from build123d import *

# Parameters (mm, degrees)
SKETCH050_R      = 14.2875
PAD049_DEPTH     = 12.7
SKETCH049_R      = 23.8125
SKETCH049_R_2    = 6.35
PAD050_DEPTH     = 25.4
CHAMFER003_SIZE2 = 11.11
CHAMFER003_SIZE  = 4.76


with BuildPart() as body048:
    # Sketch050 → Pad049 (new body)
    with BuildSketch(Plane.XZ):
        Circle(SKETCH050_R)
    extrude(amount=PAD049_DEPTH)


with BuildPart() as chamfer003:
    # Sketch049 → Pad050 (new body)
    with BuildSketch(Plane.XZ):
        Circle(SKETCH049_R)
        Circle(SKETCH049_R_2, mode=Mode.SUBTRACT)
    extrude(amount=PAD050_DEPTH)

    # Cut047: cut Body048
    add(body048.part, mode=Mode.SUBTRACT)

    # Chamfer003
    chamfer003_edges = [chamfer003.edges().sort_by_distance(p)[0] for p in [
        (-23.8125, -25.4, 0),
    ]]
    chamfer003_side = chamfer003.faces().sort_by_distance((-23.8125, -12.7, 0))[0]
    chamfer(chamfer003_edges, length=CHAMFER003_SIZE, length2=CHAMFER003_SIZE2, reference=chamfer003_side)


with BuildPart() as chamfer003_1:
    # Chamfer003 placement: moved
    add(chamfer003.part.moved(Location((0, -12.7, 0))))


solid = chamfer003_1.part
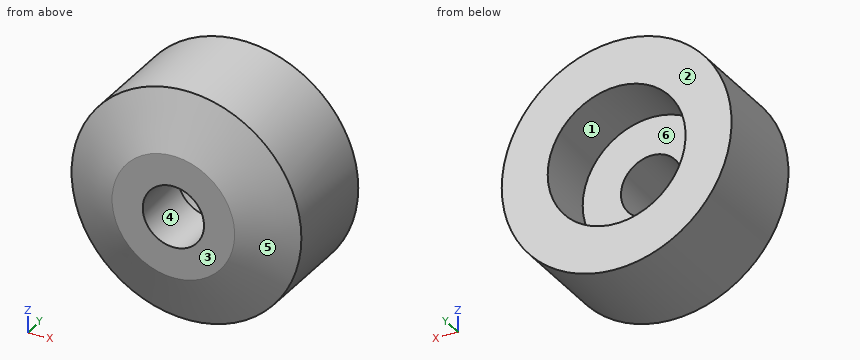
For this review, take the finished solid that the model builds, in its own axes (mm). Face numbers are marked on the shaded views. A direction names the side the tool comes from. Give positions to 0.01 mm unless a question says otherwise; leave off trailing zeros. Order: outer loops, then holes, each group sorted by start corner. A loop starts at its lowest first (then second) coordinate and runs counter-clockwise, first axis right, second up. Notation, with made-up numbers: M -16,-2 L -9,-2 A8 cw -9,5 Z; hole C -36.5,71.5 d9. An arc over 180 degrees is marked long. Answer in a Markdown table with one row per item. Add a question column.
(1) Consider section C-C on y = -22.5. State the section outline as (x, z) points (1 decimal), and give its area (3 significant figures).
(2) Wall thickness on probe 1 along Z at (x, y) = (0, -21.75); probe 2 along Z at (x, y) = (0, -29.5); probe 3 along Y at (x, z) = (-10.5, 5): over which ranges is each line inside the solid? List them lowest first. Write a range as [from, to].
(3) Consider section A-A on z = 0. State the section outline as (x, y) points, and give its area (3 significant figures).
(4) For the marked faces 1 and 2, list the 3-axis set-ups (+Z, -Z, +X, -X, +Y, -Y) from which the entire face can be reached by the end or side of a thin tool; tool diameter is ignored.
(5) Mouldability with a two-part tool opening along Z and no side actions: class the marked faces 3, 4, 5 and 6 as +Z half, -Z half, draft (parallel to the pull), parting line (faces both ways), or undercut.
(6) Consider section B-B on x = 0. State the section outline as (y, z) points.
(7) For pin 1 (1 mm diameter, centred on y = -18.5, z = 4, fed in from +X); pin 2 (12 mm diameter, centred on x = -12, y = -32, fed in from +Z); pin 3 (5 mm diameter, centred on y = -32.5, z = -9, fed in from -X), all flat-tipped, find the tip position at first contact; note any pin that passes through.
Evaluation:
| question | item | result |
|---|---|---|
| 1 | outline | C 0,0 d47.6; hole C 0,0 d28.6 |
| 1 | area | 1,140 mm^2 |
| 2 | probe 1 | z = [-23.81, -14.29], [14.29, 23.81] |
| 2 | probe 2 | z = [-23.81, -6.35], [6.35, 23.81] |
| 2 | probe 3 | y = [-38.1, -25.4] |
| 3 | outline | M -23.81,-33.34 L -12.7,-38.1 L -6.35,-38.1 L -6.35,-25.4 L -14.29,-25.4 L -14.29,-12.7 L -23.81,-12.7 Z; M 6.35,-38.1 L 12.7,-38.1 L 23.81,-33.34 L 23.81,-12.7 L 14.29,-12.7 L 14.29,-25.4 L 6.35,-25.4 Z |
| 3 | area | 633 mm^2 |
| 4 | face 1 | +Y |
| 4 | face 2 | +Z, -Z, +X, -X, +Y |
| 5 | face 3 | draft |
| 5 | face 4 | undercut |
| 5 | face 5 | parting line |
| 5 | face 6 | undercut |
| 6 | outline | M -38.1,-12.7 L -33.34,-23.81 L -12.7,-23.81 L -12.7,-14.29 L -25.4,-14.29 L -25.4,-6.35 L -38.1,-6.35 Z; M -38.1,6.35 L -25.4,6.35 L -25.4,14.29 L -12.7,14.29 L -12.7,23.81 L -33.34,23.81 L -38.1,12.7 Z |
| 7 | pin 1 | stops at x = 23.55 |
| 7 | pin 2 | stops at z = 23.04 |
| 7 | pin 3 | stops at x = -22.91 |
